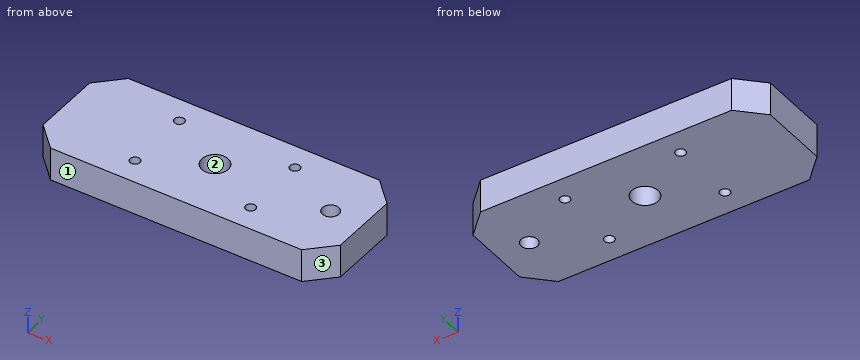
from build123d import *

# Parameters (mm, degrees)
SKETCH_1_W      = 90
SKETCH_1_H      = 35
SKETCH_1_R      = 2.5
SKETCH_1_R_2    = 4
SKETCH_1_R_3    = 1.5
EXTRUDE_1_DEPTH = 10
CHAMFER_1_SIZE  = 7


with BuildPart() as part:
    # ｽｹｯﾁ1 → ﾎﾞｽ - 押し出し1 (new body)
    with BuildSketch(Plane.XY):
        Rectangle(SKETCH_1_W, SKETCH_1_H)
        with Locations((35, 0)):
            Circle(SKETCH_1_R, mode=Mode.SUBTRACT)
        Circle(SKETCH_1_R_2, mode=Mode.SUBTRACT)
        with Locations((17.5, 10)):
            Circle(SKETCH_1_R_3, mode=Mode.SUBTRACT)
        with Locations(Location((17.5, -10, 0), (0, 0, 180))):
            Circle(SKETCH_1_R_3, mode=Mode.SUBTRACT)
        with Locations(Location((-17.5, 10, 0), (0, 0, 180))):
            Circle(SKETCH_1_R_3, mode=Mode.SUBTRACT)
        with Locations((-17.5, -10)):
            Circle(SKETCH_1_R_3, mode=Mode.SUBTRACT)
    extrude(amount=EXTRUDE_1_DEPTH)

    # 面取り1
    chamfer_1_edges = [part.edges().sort_by_distance(p)[0] for p in [
        (-45, 17.5, 5),
        (45, 17.5, 5),
        (45, -17.5, 5),
        (-45, -17.5, 5),
    ]]
    chamfer(chamfer_1_edges, length=CHAMFER_1_SIZE)


solid = part.part
Could you check a few things on this model? Use its own coordinates, in mm. Face numbers are marked on the shaded views. Give positions to 0.01 mm unless a question says otherwise; leave off trailing zeros. Order: outer loops, then holes, each group sorted by start corner. A loop starts at its lowest first (then second) coordinate and runs counter-clockwise, first axis right, second up.
Item 1: If we mould it in two halves opening along X, with no side actions, what happens to the marked faces 1, 2 and 3? For each: pulls with the +X half, pulls with the -X half, needs draft (parallel to the pull), parting line crosses it, or undercut.
Item 2: If we section it at D-D, the plane z = 2.75: Write out the boundary of the cut face in (x, y), plus the area to 3 significant figures.
Item 3: I need wall thicknesses on line 1 (Y direction, x = 17.5, z = 3.5); line 2 (X direction, y = -1.5, z = 1.5); line 3 (X direction, y = 10.5, z = 1.5). Which ranges of each line are inside material? Lowest first, please.
Item 4: If we section it at A-A, the plane x = -17.5: Write out the boundary of the cut face in (y, z).
Item 5: If we section it at C-C, the plane x = 35: Write out the boundary of the cut face in (y, z).
Item 6: If we section it at B-B, the plane y = 0: Write out the boundary of the cut face in (x, z).
Values:
1. face 1: needs draft
1. face 2: undercut
1. face 3: pulls with the +X half
2. outline: (-45, -10.5) - (-38, -17.5) - (38, -17.5) - (45, -10.5) - (45, 10.5) - (38, 17.5) - (-38, 17.5) - (-45, 10.5) - close; hole circle Ø3 at (-17.5, -10); hole circle Ø3 at (-17.5, 10); hole circle Ø8 at (0, 0); hole circle Ø3 at (17.5, -10); hole circle Ø3 at (17.5, 10); hole circle Ø5 at (35, 0)
2. area: 2,950 mm2
3. line 1: y = -17.5 to -11.5, -8.5 to 8.5, 11.5 to 17.5
3. line 2: x = -45 to -3.71, 3.71 to 33, 37 to 45
3. line 3: x = -45 to -18.91, -16.09 to 16.09, 18.91 to 45
4. outline: (-17.5, 0) - (-11.5, 0) - (-11.5, 10) - (-17.5, 10) - close; (-8.5, 0) - (8.5, 0) - (8.5, 10) - (-8.5, 10) - close; (11.5, 0) - (17.5, 0) - (17.5, 10) - (11.5, 10) - close
5. outline: (-17.5, 0) - (-2.5, 0) - (-2.5, 10) - (-17.5, 10) - close; (2.5, 0) - (17.5, 0) - (17.5, 10) - (2.5, 10) - close
6. outline: (-45, 0) - (-4, 0) - (-4, 10) - (-45, 10) - close; (4, 0) - (32.5, 0) - (32.5, 10) - (4, 10) - close; (37.5, 0) - (45, 0) - (45, 10) - (37.5, 10) - close
